```python
from build123d import *

# Parameters (mm, degrees)
BOX252_W          = 40
BOX252_H          = 20
BOX252_DEPTH      = 40
CYLINDER650_R     = 4.1
CYLINDER650_DEPTH = 10
CYLINDER649_R     = 8
CYLINDER649_DEPTH = 8


with BuildPart() as krychle252:
    # Box252 → Box252 (new body)
    with BuildSketch(Plane(origin=(-20, 110, 30), x_dir=(1, 0, 0), z_dir=(0, 0, 1))):
        with Locations((20, 10)):
            Rectangle(BOX252_W, BOX252_H)
    extrude(amount=BOX252_DEPTH)


with BuildPart() as obj1:
    # Cylinder650 → Cylinder650 (new body)
    with BuildSketch(Plane(origin=(0, 118, 50), x_dir=(1, 0, 0), z_dir=(0, -1, 0))):
        Circle(CYLINDER650_R)
    extrude(amount=CYLINDER650_DEPTH)


with BuildPart() as cut260:
    # Cylinder649 → Cylinder649 (new body)
    with BuildSketch(Plane(origin=(0, 114, 50), x_dir=(1, 0, 0), z_dir=(0, -1, 0))):
        Circle(CYLINDER649_R)
    extrude(amount=CYLINDER649_DEPTH)

    # Cut255: cut obj1
    add(obj1.part, mode=Mode.SUBTRACT)

    # Cut260: cut Krychle252
    add(krychle252.part, mode=Mode.SUBTRACT)


solid = cut260.part
```
Read the model definition and answer for the solid it produces. Units are mm, in the model's axes. A direction names the side the tool comes from. Coordinates: 2 decimals unless noted, no trailing zeros. Loops run counter-clockwise (first coordinate to the right, second up) from the corner with the lowest first, then second, coordinate; pieces in that order, holes last.
(1) The mould has two halves that part along Z. Classify faces 3 (the face through (0, 106, 50)), 4 (the face through (-1.041, 108.028, 57.932)), 5 (the face through (0, 108, 50)): released by +Z, released by -Z, zero draft, split by the parting line, or undercut.
Solution:
face 3: zero draft
face 4: split by the parting line
face 5: undercut
(2) The part is cut by section D-D (y = 106.3). Determine the outline of the cut face in (x, z).
Solution:
outline: circle Ø16 at (0, 50)
(3) The part is cut by section A-A (x = 0). Determine the outline of the cut face in (y, z), and give its area (3 significant figures).
Solution:
outline: (106, 42) - (110, 42) - (110, 45.9) - (108, 45.9) - (108, 54.1) - (110, 54.1) - (110, 58) - (106, 58) - close
area: 47.6 mm2
(4) Consider line 1 along X through (y, z) = (109.2, 50); line 2 along Z through (x, y) = (0, 109.05); line 3 along Y through (x, z) = (-3.25, 48.25). Determine where each line is inside the solid, lowest interval first.
Solution:
line 1: x = -8 to -4.1, 4.1 to 8
line 2: z = 42 to 45.9, 54.1 to 58
line 3: y = 106 to 108
(5) The part is cut by section C-C (z = 50). Determine the outline of the cut face in (x, y).
Solution:
outline: (-8, 106) - (8, 106) - (8, 110) - (4.1, 110) - (4.1, 108) - (-4.1, 108) - (-4.1, 110) - (-8, 110) - close
(6) A tool of negligible diameter and unlimited length cuts with its end or side. For faces 1 (the face through (-3.022, 109.014, 52.771)), 2 (the face through (-2, 110, 46)), from which of +Z, -Z, +X, -X, +Y, -Y can it reach the whole face along a straight path? Write none if from no direction.
Solution:
face 1: +Y
face 2: +Z, -Z, +X, -X, +Y
(7) The part is cut by section B-B (y = 109.45). Determine the outline of the cut face in (x, z).
Solution:
outline: circle Ø16 at (0, 50); hole circle Ø8.2 at (0, 50)
(8) A flat-ended cylindrical pin translates along its axis: pin 1 Ø1 at (x, y) = (-4.5, 107.5) entering from -Z. Find the tip coordinate at first contact, or state that the pin passes through.
Solution:
pin 1: stops at z = 43.07
